```python
from build123d import *

# Parameters (mm, degrees)
F0_W            = 64
F0_H            = 64
F1_DEPTH        = 10
F3_DEPTH        = 64.001
F4_W            = 20
F4_H            = 34.5
F5_W            = 3
F5_H            = 26.7061145455
F5_W_2          = 10
F6_DEPTH        = 7.6
F7_R            = 4.5
F8_DEPTH        = 64.001
F10_DEPTH       = 10
F11_W           = 20
F11_H           = 40
F12_DEPTH       = 10
F13_W           = 20
F13_H           = 12
F14_DEPTH       = 7
F16_DEPTH       = 20.001
F18_D           = 2.5
F18_DEPTH       = 4
F18_TIP         = 0.7510757738
F20_D           = 2.5
F20_DEPTH       = 4
F20_CBORE_D     = 3.5
F20_CBORE_DEPTH = 3.5
F20_TIP         = 0.7510757738
F21_W           = 0.75
F21_H           = 0.25
F21_H_2         = 2.25
F21_H_3         = 0.75
F21_H_4         = 2.5
F22_DEPTH       = 6
F23_W           = 3
F23_H           = 1.5
F23_W_2         = 1.5
F24_DEPTH       = 10
F25_W           = 3
F25_H           = 16
F26_DEPTH       = 2


with BuildPart() as f1:
    # F0 (on Top) → F1 (new body)
    with BuildSketch(Plane.XY):
        with Locations((32, 32)):
            Rectangle(F0_W, F0_H)
    extrude(amount=F1_DEPTH)

    # F2 (on face) → F3 (cut, through all)
    with BuildSketch(Plane.YZ.offset(64)):
        with BuildLine():
            Line((14.5, 0), (29.5, 0))
            ThreePointArc((29.5, 0), (22, 7.5), (14.5, 0))
        make_face()
        with BuildLine():
            ThreePointArc((59.5, 0), (52, 7.5), (44.5, 0))
            Line((44.5, 0), (59.5, 0))
        make_face()
    extrude(amount=-F3_DEPTH, mode=Mode.SUBTRACT)

    # F4 (on face) + F5 (on face) → F6 (join)
    with BuildSketch(Plane(origin=(0, 0, 0), x_dir=(1, 0, 0), z_dir=(0, 0, -1))):
        with Locations((10, -17.25)):
            Rectangle(F4_W, F4_H)
        with Locations((54, -17.25)):
            Rectangle(F4_W, F4_H)
    with BuildSketch(Plane(origin=(0, 0, 0), x_dir=(1, 0, 0), z_dir=(0, 0, -1))):
        with Locations((1.5, -50.6469427273)):
            Rectangle(F5_W, F5_H)
        with Locations((32, -50.6469427273)):
            Rectangle(F5_W_2, F5_H)
        with Locations((62.5, -50.6469427273)):
            Rectangle(F5_W, F5_H)
    extrude(amount=-F6_DEPTH)

    # F7 (on face) → F8 (cut, through all)
    with BuildSketch(Plane(origin=(0, 0, 0), x_dir=(0, -1, 0), z_dir=(-1, 0, 0))):
        with Locations((-52, 0)):
            Circle(F7_R)
        with Locations((-22, 0)):
            Circle(F7_R)
    extrude(amount=-F8_DEPTH, mode=Mode.SUBTRACT)

    # F9 (on face) → F10 (join)
    with BuildSketch(Plane.XY.offset(10)):
        Polygon((18, 44), (18, 0), (58, 0), (58, 10), (46, 10), (46, 44), align=None)
    extrude(amount=F10_DEPTH)

    # F11 (on face) → F12 (cut)
    with BuildSketch(Plane.XY.offset(20)):
        with Locations((32, 20)):
            Rectangle(F11_W, F11_H)
    extrude(amount=-F12_DEPTH, mode=Mode.SUBTRACT)

    # F13 (on face) → F14 (cut)
    with BuildSketch(Plane.XY.offset(10)):
        with Locations((32, 6)):
            Rectangle(F13_W, F13_H)
    extrude(amount=-F14_DEPTH, mode=Mode.SUBTRACT)

    # F15 (on face) → F16 (cut, through all)
    with BuildSketch(Plane.XY.offset(20)):
        Polygon((47, 0), (50, 0), (50, 4), (45, 4), align=None)
        Polygon((50, 4), (50, 0), (53, 0), (55, 4), align=None)
    extrude(amount=-F16_DEPTH, mode=Mode.SUBTRACT)

    # F18
    with Locations(Plane.XZ.offset(-12)):
        with Locations((27, 5.5), (37, 5.5)):
            Hole(F18_D / 2, depth=F18_DEPTH)
            with Locations((0, 0, -(F18_DEPTH + F18_TIP / 2))):  # 118° drill point
                Cone(0, F18_D / 2, F18_TIP, mode=Mode.SUBTRACT)

    # F20
    with Locations(Plane(origin=(0, 44, 0), x_dir=(-1, 0, 0), z_dir=(0, 1, 0))):
        with Locations((-39.5, 12), (-24.5, 12)):
            CounterBoreHole(F20_D / 2, F20_CBORE_D / 2, F20_CBORE_DEPTH, depth=F20_DEPTH)
            with Locations((0, 0, -(F20_DEPTH + F20_TIP / 2))):  # 118° drill point
                Cone(0, F20_D / 2, F20_TIP, mode=Mode.SUBTRACT)

    # F21 (on face) → F22 (cut)
    with BuildSketch(Plane.XY.offset(10)):
        with Locations((9.625, 32.125)):
            Rectangle(F21_W, F21_H)
        with BuildLine():
            Line((53.25, 33), (53.25, 32))
            Line((53.25, 32), (54, 32))
            Line((54, 32), (54, 32.25))
            ThreePointArc((54, 32.25), (53.4696699141, 32.4696699141), (53.25, 33))
        make_face()
        with BuildLine():
            Line((54, 32), (53.25, 32))
            Line((53.25, 32), (53.25, 29))
            ThreePointArc((53.25, 29), (53.4696699141, 29.5303300859), (54, 29.75))
            Line((54, 29.75), (54, 32))
        make_face()
        with Locations((9.625, 30.875)):
            Rectangle(F21_W, F21_H_2)
        with BuildLine():
            Line((10, 32.25), (10, 32))
            Line((10, 32), (10.75, 32))
            Line((10.75, 32), (10.75, 33))
            ThreePointArc((10.75, 33), (10.5303300859, 32.4696699141), (10, 32.25))
        make_face()
        with BuildLine():
            Line((10.75, 32), (10, 32))
            Line((10, 32), (10, 29.75))
            ThreePointArc((10, 29.75), (10.5303300859, 29.5303300859), (10.75, 29))
            Line((10.75, 29), (10.75, 32))
        make_face()
        with BuildLine():
            Line((0, 32.25), (9.25, 32.25))
            Line((9.25, 32.25), (9.25, 33))
            ThreePointArc((9.25, 33), (9.4696699141, 33.5303300859), (10, 33.75))
            Line((10, 33.75), (0, 33.75))
            ThreePointArc((0, 33.75), (-0.75, 33), (0, 32.25))
        make_face()
        with Locations((9.625, 32.625)):
            Rectangle(F21_W, F21_H_3)
        with Locations((9.625, 29.375)):
            Rectangle(F21_W, F21_H_3)
        with BuildLine():
            Line((9.25, 29), (9.25, 29.75))
            Line((9.25, 29.75), (0, 29.75))
            ThreePointArc((0, 29.75), (-0.75, 29), (0, 28.25))
            Line((0, 28.25), (10, 28.25))
            ThreePointArc((10, 28.25), (9.4696699141, 28.4696699141), (9.25, 29))
        make_face()
        with BuildLine():
            Line((10, 33), (10, 32.25))
            ThreePointArc((10, 32.25), (10.5303300859, 32.4696699141), (10.75, 33))
            ThreePointArc((10.75, 33), (10.5303300859, 33.5303300859), (10, 33.75))
            ThreePointArc((10, 33.75), (9.4696699141, 33.5303300859), (9.25, 33))
            Line((9.25, 33), (10, 33))
        make_face()
        with BuildLine():
            ThreePointArc((10.75, 29), (10.5303300859, 29.5303300859), (10, 29.75))
            Line((10, 29.75), (10, 29))
            Line((10, 29), (9.25, 29))
            ThreePointArc((9.25, 29), (9.4696699141, 28.4696699141), (10, 28.25))
            ThreePointArc((10, 28.25), (10.5303300859, 28.4696699141), (10.75, 29))
        make_face()
        with Locations((54.375, 32.125)):
            Rectangle(F21_W, F21_H)
        with Locations((54.375, 30.875)):
            Rectangle(F21_W, F21_H_2)
        with BuildLine():
            ThreePointArc((54, 33.75), (53.4696699141, 33.5303300859), (53.25, 33))
            ThreePointArc((53.25, 33), (53.4696699141, 32.4696699141), (54, 32.25))
            Line((54, 32.25), (54, 33))
            Line((54, 33), (54.75, 33))
            ThreePointArc((54.75, 33), (54.5303300859, 33.5303300859), (54, 33.75))
        make_face()
        with BuildLine():
            ThreePointArc((54, 29.75), (53.4696699141, 29.5303300859), (53.25, 29))
            ThreePointArc((53.25, 29), (53.4696699141, 28.4696699141), (54, 28.25))
            ThreePointArc((54, 28.25), (54.5303300859, 28.4696699141), (54.75, 29))
            Line((54.75, 29), (54, 29))
            Line((54, 29), (54, 29.75))
        make_face()
        with Locations((54.375, 32.625)):
            Rectangle(F21_W, F21_H_3)
        with Locations((54.375, 29.375)):
            Rectangle(F21_W, F21_H_3)
        with BuildLine():
            Line((64, 33.75), (54, 33.75))
            ThreePointArc((54, 33.75), (54.5303300859, 33.5303300859), (54.75, 33))
            Line((54.75, 33), (54.75, 32.25))
            Line((54.75, 32.25), (64, 32.25))
            ThreePointArc((64, 32.25), (64.75, 33), (64, 33.75))
        make_face()
        with BuildLine():
            ThreePointArc((54.75, 29), (54.5303300859, 28.4696699141), (54, 28.25))
            Line((54, 28.25), (64, 28.25))
            ThreePointArc((64, 28.25), (64.75, 29), (64, 29.75))
            Line((64, 29.75), (54.75, 29.75))
            Line((54.75, 29.75), (54.75, 29))
        make_face()
        with BuildLine():
            ThreePointArc((10, 39.75), (9.4696699141, 39.5303300859), (9.25, 39))
            Line((9.25, 39), (10, 39))
            Line((10, 39), (10, 38.25))
            ThreePointArc((10, 38.25), (10.5303300859, 38.4696699141), (10.75, 39))
            ThreePointArc((10.75, 39), (10.5303300859, 39.5303300859), (10, 39.75))
        make_face()
        with BuildLine():
            Line((9.25, 38.25), (9.25, 39))
            ThreePointArc((9.25, 39), (9.4696699141, 39.5303300859), (10, 39.75))
            Line((10, 39.75), (0, 39.75))
            ThreePointArc((0, 39.75), (-0.75, 39), (0, 38.25))
            Line((0, 38.25), (9.25, 38.25))
        make_face()
        with Locations((9.625, 38.625)):
            Rectangle(F21_W, F21_H_3)
        with Locations((9.625, 37)):
            Rectangle(F21_W, F21_H_4)
        with BuildLine():
            ThreePointArc((10.75, 39), (10.5303300859, 38.4696699141), (10, 38.25))
            Line((10, 38.25), (10, 35.75))
            ThreePointArc((10, 35.75), (10.5303300859, 35.5303300859), (10.75, 35))
            Line((10.75, 35), (10.75, 39))
        make_face()
        with BuildLine():
            Line((9.25, 35), (9.25, 35.75))
            Line((9.25, 35.75), (0, 35.75))
            ThreePointArc((0, 35.75), (-0.75, 35), (0, 34.25))
            Line((0, 34.25), (10, 34.25))
            ThreePointArc((10, 34.25), (9.4696699141, 34.4696699141), (9.25, 35))
        make_face()
        with Locations((9.625, 35.375)):
            Rectangle(F21_W, F21_H_3)
        with BuildLine():
            ThreePointArc((10.75, 35), (10.5303300859, 35.5303300859), (10, 35.75))
            Line((10, 35.75), (10, 35))
            Line((10, 35), (9.25, 35))
            ThreePointArc((9.25, 35), (9.4696699141, 34.4696699141), (10, 34.25))
            ThreePointArc((10, 34.25), (10.5303300859, 34.4696699141), (10.75, 35))
        make_face()
        with Locations((54.375, 35.375)):
            Rectangle(F21_W, F21_H_3)
        with BuildLine():
            Line((54.75, 35), (54, 35))
            Line((54, 35), (54, 35.75))
            ThreePointArc((54, 35.75), (53.4696699141, 35.5303300859), (53.25, 35))
            ThreePointArc((53.25, 35), (53.4696699141, 34.4696699141), (54, 34.25))
            ThreePointArc((54, 34.25), (54.5303300859, 34.4696699141), (54.75, 35))
        make_face()
        with BuildLine():
            Line((54.75, 35.75), (54.75, 35))
            ThreePointArc((54.75, 35), (54.5303300859, 34.4696699141), (54, 34.25))
            Line((54, 34.25), (64, 34.25))
            ThreePointArc((64, 34.25), (64.75, 35), (64, 35.75))
            Line((64, 35.75), (54.75, 35.75))
        make_face()
        with BuildLine():
            ThreePointArc((53.25, 35), (53.4696699141, 35.5303300859), (54, 35.75))
            Line((54, 35.75), (54, 38.25))
            ThreePointArc((54, 38.25), (53.4696699141, 38.4696699141), (53.25, 39))
            Line((53.25, 39), (53.25, 35))
        make_face()
        with Locations((54.375, 37)):
            Rectangle(F21_W, F21_H_4)
        with BuildLine():
            ThreePointArc((53.25, 39), (53.4696699141, 38.4696699141), (54, 38.25))
            Line((54, 38.25), (54, 39))
            Line((54, 39), (54.75, 39))
            ThreePointArc((54.75, 39), (54.5303300859, 39.5303300859), (54, 39.75))
            ThreePointArc((54, 39.75), (53.4696699141, 39.5303300859), (53.25, 39))
        make_face()
        with Locations((54.375, 38.625)):
            Rectangle(F21_W, F21_H_3)
        with BuildLine():
            Line((54.75, 39), (54.75, 38.25))
            Line((54.75, 38.25), (64, 38.25))
            ThreePointArc((64, 38.25), (64.75, 39), (64, 39.75))
            Line((64, 39.75), (54, 39.75))
            ThreePointArc((54, 39.75), (54.5303300859, 39.5303300859), (54.75, 39))
        make_face()
    extrude(amount=-F22_DEPTH, mode=Mode.SUBTRACT)

    # F23 (on face) → F24 (cut, through all)
    with BuildSketch(Plane(origin=(0, 0, 0), x_dir=(1, 0, 0), z_dir=(0, 0, -1))):
        with Locations((49, -43.25)):
            Rectangle(F23_W, F23_H)
        with Locations((49, -60.75)):
            Rectangle(F23_W, F23_H)
        with Locations((14.25, -60.75)):
            Rectangle(F23_W_2, F23_H)
        with Locations((15.75, -60.75)):
            Rectangle(F23_W_2, F23_H)
        with Locations((15, -43.25)):
            Rectangle(F23_W, F23_H)
        with Locations((32.75, -30.75)):
            Rectangle(F23_W_2, F23_H)
        with Locations((31.25, -30.75)):
            Rectangle(F23_W_2, F23_H)
        with Locations((32, -13.25)):
            Rectangle(F23_W, F23_H)
    extrude(amount=-F24_DEPTH, mode=Mode.SUBTRACT)

    # F25 (on face) → F26 (cut)
    with BuildSketch(Plane.XY.offset(10)):
        with Locations((32, 22)):
            Rectangle(F25_W, F25_H)
    extrude(amount=-F26_DEPTH, mode=Mode.SUBTRACT)


solid = f1.part
```
Work out the finished part from the listing and answer in its coordinate system (mm). A direction names the side the tool comes from. Give positions to 0.01 mm unless a question says otherwise; leave off trailing zeros. Loops run counter-clockwise (first coordinate to the right, second up) from the corner with the lowest first, then second, coordinate; pieces in that order, holes last. Notation, with made-up numbers: (25.25, 11) -> (30.25, 11) arc R32 cw to (30.25, 44) -> close; hole circle Ø8 at (11, -33). An arc over 180 degrees is marked (long way). Put each result on its own line as item: value. Start each with the question number.
Item 1: The part is cut by section A-A (x = 15.5). Give the vertices of the cut face in (y, z), then the cut area to 3 significant figures.
Item 2: The part is cut by section C-C (x = 24.5). Give the vertices of the cut face in (y, z), then the cut area to 3 significant figures.
Item 3: The part is cut by section B-B (z = 15.5). Give the vertices of the cut face in (x, y), then the cut area to 3 significant figures.
Item 4: Each of these flat-tipped pins is pushed along its axis until it touches: P1, Ø4, axis at x = 21.5, z = 14, coming from the +Y side; P2, Ø0.8, axis at y = 60.5, z = 3.5, coming from the -X side; P3, Ø6, axis at x = 28, z = 6.5, coming from the -Y side; P4, Ø2, axis at x = 59, y = 31, coming from the +Z side. Where does it stop, or does it pass through?
Item 5: The part is cut by section D-D (y = 49). Give the vertices of the cut face in (x, z).
Item 6: Which of the six approach directions +Z, -Z, +X, -X, +Y, -Y give full straight-line access (tool end or side, diameter ignored) to faces 1 (the face through (46, 27, 15)), 2 (the face through (5, 34.25, 7)), 3 (the face through (49, 60, 5)), 4 (the face through (26, 40.5, 12)), 5 (the face through (59, 32.25, 7))?
Item 7: The mould has two halves that part along X. Classify faces 6 (the face through (49.17, 52.16, 7.5)), 7 (the face through (5, 32.25, 7)), 8 (the face through (64, 32, 5)): released by +X, released by -X, zero draft, split by the parting line, or undercut.
Item 8: Find the intervals of material crossed by L1, parallel to X at y = 43, z = 2.75; L2, parallel to X at y = 40.35, z = 12; L3, parallel to Y at x = 61, z = 8.25, in increasing order. Write a range as [from, to].
Answers below:
1. outline: (0, 0) -> (17.5, 0) arc R4.5 cw to (26.5, 0) -> (42.5, 0) -> (42.5, 10) -> (0, 10) -> close; (44, 0) -> (44.5, 0) arc R7.5 cw to (59.5, 0) -> (60, 0) -> (60, 10) -> (44, 10) -> close; (61.5, 0) -> (64, 0) -> (64, 10) -> (61.5, 10) -> close
1. area: 490 mm2
2. outline: (0, 0) -> (14.5, 0) arc R7.5 cw to (29.5, 0) -> (44.5, 0) arc R7.5 cw to (59.5, 0) -> (64, 0) -> (64, 10) -> (44, 10) -> (44, 10.25) -> (40.5, 10.25) -> (40.5, 10.75) -> (40, 10.75) -> (40, 10) -> (12, 10) -> (12, 3) -> (0, 3) -> close; (40, 13.25) -> (40.5, 13.25) -> (40.5, 13.75) -> (44, 13.75) -> (44, 20) -> (40, 20) -> close
2. area: 406 mm2
3. outline: (18, 0) -> (22, 0) -> (22, 40) -> (42, 40) -> (42, 0) -> (47, 0) -> (45, 4) -> (55, 4) -> (53, 0) -> (58, 0) -> (58, 10) -> (46, 10) -> (46, 44) -> (18, 44) -> close
3. area: 520 mm2
4. P1: y = 44
4. P2: x = 0
4. P3: y = 12
4. P4: z = 10
5. outline: (0, 3.35) -> (3, 3.35) -> (3, 6.87) -> (27, 6.87) -> (27, 3.35) -> (37, 3.35) -> (37, 6.87) -> (61, 6.87) -> (61, 3.35) -> (64, 3.35) -> (64, 10) -> (0, 10) -> close
6. face 1: +Z, +X, +Y
6. face 2: +Z, -X
6. face 3: +Z, -Z
6. face 4: +Y
6. face 5: +Z, +X
7. face 6: undercut
7. face 7: zero draft
7. face 8: released by +X
8. L1: [0, 13.5], [16.5, 47.5], [50.5, 64]
8. L2: [18, 23.25], [25.75, 38.25], [40.75, 46]
8. L3: [0, 28.25], [29.75, 32.25], [33.75, 34.25], [35.75, 38.25], [39.75, 64]
